Input: dimensioned drawing with shaded views. Units: mm. Origin: part minimum x, y, z. Round coordinates to 2 decimals unless told otherwise and drop trailing zeros. Loops run counter-clockwise (first coordinate to the right, second up) from the corner with the lowest first, then second, coordinate; pieces in that order, holes last. Notation, with made-up numbers: (-39.5, 47) - (-19.5, 47) arc R10 cw to (-19.5, 58) - close; hole circle Ø7 at (-26.75, 88.25). An arc over 180 degrees is marked (long way). One line per question, with ' | ' between items. Start each with the question number.
Item 1: Section C-C, the plane y = 35.32. Return loops of the section in (x, z).
Item 2: Section B-B, the plane z = 1. Return loops of the section in (x, y).
Item 3: Section A-A, the plane x = 16.5. Return loops of the section in (y, z).
Item 4: Material intervals for line 1 along X through (y, z) = (43, 0.15); line 2 along X through (y, z) = (35.5, 1.7); line 3 along Y through (x, z) = (39.71, 0.6), sorted ascending.
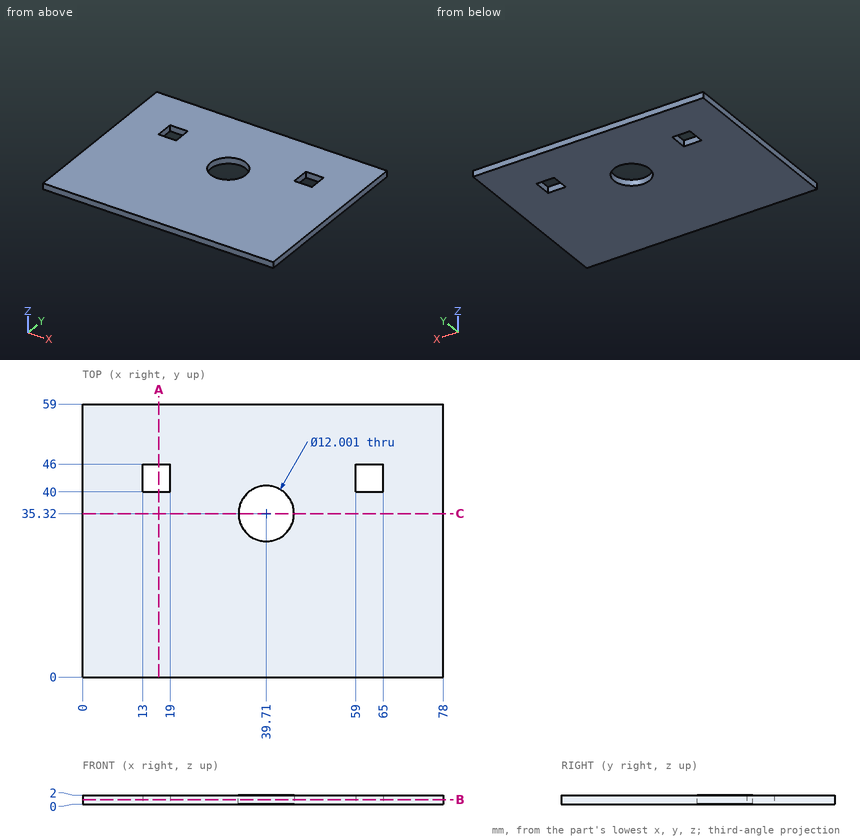
Return value:
1) outline: (0, 0) - (33.71, 0) - (33.71, 2) - (0, 2) - close; (45.71, 0) - (78, 0) - (78, 2) - (45.71, 2) - close
2) outline: (0, 0) - (78, 0) - (78, 59) - (0, 59) - close; hole (13, 40) - (19, 40) - (19, 46) - (13, 46) - close; hole circle Ø12 at (39.71, 35.32); hole (59, 40) - (65, 40) - (65, 46) - (59, 46) - close
3) outline: (0, 0) - (40, 0) - (40, 2) - (0, 2) - close; (46, 0) - (59, 0) - (59, 2) - (46, 2) - close
4) line 1: 0 to 13, 19 to 59, 65 to 78 | line 2: 0 to 33.71, 45.71 to 78 | line 3: 0 to 29.32, 41.32 to 59
